```python
from build123d import *

# Parameters (mm, degrees)
SKETCH1_W           = 39.7
SKETCH1_H           = 39.7
BOSS_EXTRUDE1_DEPTH = 7.5
SKETCH2_W           = 35.8
SKETCH2_H           = 21.8
BOSS_EXTRUDE2_DEPTH = 2.8
SHELL1_T            = -0.5
SKETCH4_W           = 1
SKETCH4_H           = 1
BOSS_EXTRUDE3_DEPTH = 5
SKETCH5_W           = 1
SKETCH5_H           = 1
BOSS_EXTRUDE4_DEPTH = 5
SKETCH6_W           = 38.7
SKETCH6_H           = 15.557355087
BOSS_EXTRUDE5_DEPTH = 0.1


with BuildPart() as part:
    # Sketch1 → Boss-Extrude1 (new body)
    with BuildSketch(Plane.XY):
        Rectangle(SKETCH1_W, SKETCH1_H)
    extrude(amount=BOSS_EXTRUDE1_DEPTH)

    # Sketch2 → Boss-Extrude2 (add)
    with BuildSketch(Plane.XY.offset(7.5)):
        with Locations((0, 7.15)):
            Rectangle(SKETCH2_W, SKETCH2_H)
    extrude(amount=BOSS_EXTRUDE2_DEPTH)

    # Shell1
    shell1_openings = [part.faces().sort_by_distance(p)[0] for p in [
        (0, 0, 0),
    ]]
    offset(amount=SHELL1_T, openings=shell1_openings, kind=Kind.INTERSECTION)

    # Sketch4 → Boss-Extrude3 (add)
    with BuildSketch(Plane(origin=(0, 0, 7), x_dir=(-1, 0, 0), z_dir=(0, 0, -1))):
        with Locations((-11, 18.85)):
            Rectangle(SKETCH4_W, SKETCH4_H)
        with Locations((11, 18.85)):
            Rectangle(SKETCH4_W, SKETCH4_H)
    boss_extrude3 = extrude(amount=BOSS_EXTRUDE3_DEPTH)

    # Mirror1: Boss-Extrude3 across plane
    add(boss_extrude3.mirror(Plane.ZX))

    # Sketch5 → Boss-Extrude4 (add)
    with BuildSketch(Plane(origin=(0, 0, 7), x_dir=(-1, 0, 0), z_dir=(0, 0, -1))):
        with Locations((-18.85, -7.35)):
            Rectangle(SKETCH5_W, SKETCH5_H)
        with Locations((18.85, -7.35)):
            Rectangle(SKETCH5_W, SKETCH5_H)
    extrude(amount=BOSS_EXTRUDE4_DEPTH)

    # Sketch6 → Boss-Extrude5 (add)
    with BuildSketch(Plane(origin=(0, 0, 7), x_dir=(-1, 0, 0), z_dir=(0, 0, -1))):
        with Locations((0, -11.571322457)):
            Rectangle(SKETCH6_W, SKETCH6_H)
    extrude(amount=BOSS_EXTRUDE5_DEPTH)


solid = part.part
```
Could you check a few things on this model? Use its own coordinates, in mm. A direction names the side the tool comes from. Give positions to 0.01 mm unless a question says otherwise; leave off trailing zeros. Loops run counter-clockwise (first coordinate to the right, second up) from the corner with the lowest first, then second, coordinate; pieces in that order, holes last. Notation, with made-up numbers: (-37.75, 18) - (-27.75, 18) arc R35 cw to (-27.75, 56) - close; hole circle Ø2 at (60, 75.25). An arc over 180 degrees is marked (long way). Answer in a Markdown table with one row per item. Add a question column.
Q1. If we section it at A-A (z = 8.5): List the corners of the cut face in (x, y) for me.
Q2. If we section it at B-B (y = -12): List the corners of the cut face in (x, z) for me, plus the area to 3 significant figures.
Q3. Please list where these lines run through material, in increasing order: L1, parallel to X at y = 18.5, z = 1.25; L2, parallel to Y at x = 17, z = 9.25. Write a range as from..to.
Q4. Which directions (+Z, -Z, +X, -X, +Y, -Y) give clear straight access to the entire face, cutting with the end or side of a thin tool? Please do faces 4 (the face through (11, 19, 2)), 5 (the face through (0, 7, 10.3)), 6 (the face through (17.9, 7, 9)).
Q5. If we section it at D-D (z = 1.25): List the corners of the cut face in (x, y) for me.
Q6. If we section it at C-C (x = -7.5): List the corners of the cut face in (y, z) for me.
Q7. For pin 1 (2 mm diameter, centred on x = -15, y = -8, fed in from -Z); pin 2 (1.4 mm diameter, centred on y = 4.5, z = 8.5, fed in from +X); pin 3 (2 mm diameter, centred on y = 3.5, z = 9.5, fed in from -X), each with a flat end and sliding along its axis, tell me the tip position at first contact or that it passes through.
Q8. We'd pull the mould along Y, two halves only. Please class faces 1 (the face through (0, -3.75, 9)), 2 (the face through (-19.85, 0, 4)), 3 (the face through (11.5, -19, 4)): +Y half, -Y half, draft (parallel to the pull), parting line (faces both ways), or undercut.
The answers:
| question | item | result |
|---|---|---|
| 1 | outline | (-17.9, -3.75) - (17.9, -3.75) - (17.9, 18.05) - (-17.9, 18.05) - close; hole (-17.4, -3.25) - (17.4, -3.25) - (17.4, 17.55) - (-17.4, 17.55) - close |
| 2 | outline | (-19.85, 0) - (-19.35, 0) - (-19.35, 6.9) - (19.35, 6.9) - (19.35, 0) - (19.85, 0) - (19.85, 7.5) - (-19.85, 7.5) - close |
| 2 | area | 30.7 mm^2 |
| 3 | L1 | x = -19.85..-19.35, 19.35..19.85 |
| 3 | L2 | y = -3.75..-3.25, 17.55..18.05 |
| 4 | face 4 | -Z |
| 4 | face 5 | +Z, +X, -X, +Y, -Y |
| 4 | face 6 | +Z, +X, +Y, -Y |
| 5 | outline | (-19.85, -19.85) - (19.85, -19.85) - (19.85, 19.85) - (-19.85, 19.85) - close; hole (-19.35, -19.35) - (19.35, -19.35) - (19.35, 19.35) - (-19.35, 19.35) - close |
| 6 | outline | (-19.85, 0) - (-19.35, 0) - (-19.35, 6.9) - (-3.79, 6.9) - (-3.79, 7) - (-3.25, 7) - (-3.25, 9.8) - (17.55, 9.8) - (17.55, 7) - (19.35, 7) - (19.35, 0) - (19.85, 0) - (19.85, 7.5) - (18.05, 7.5) - (18.05, 10.3) - (-3.75, 10.3) - (-3.75, 7.5) - (-19.85, 7.5) - close |
| 7 | pin 1 | stops at z = 6.9 |
| 7 | pin 2 | stops at x = 17.9 |
| 7 | pin 3 | stops at x = -17.9 |
| 8 | face 1 | -Y half |
| 8 | face 2 | draft |
| 8 | face 3 | undercut |
